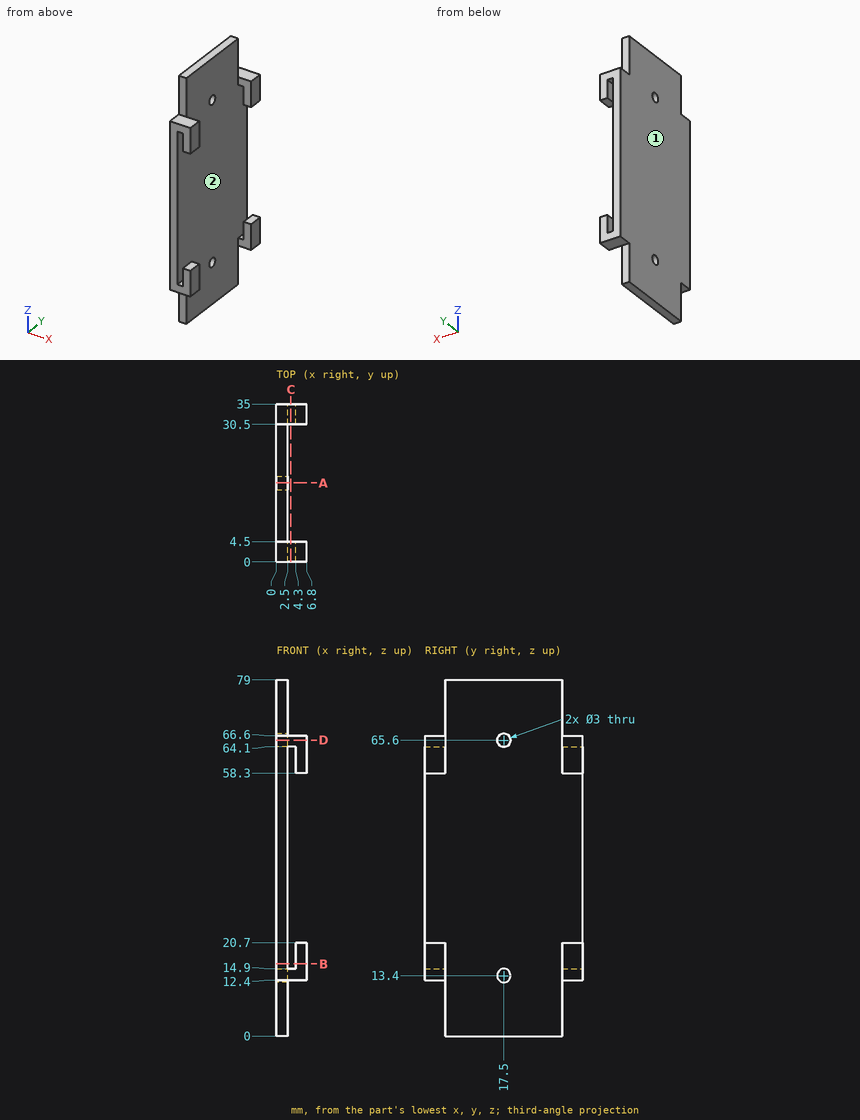
Verification items for this drawing (mm, ordinates from the low corner). Give positions to 0.01 mm unless a question says otherwise; leave off trailing zeros. Loops run counter-clockwise (first coordinate to the right, second up) from the corner with the lowest first, then second, coordinate; pieces in that order, holes last.
1. Cross-section at B-B on z = 16. Record the cut outline in (x, y).
Derived:
outline: (0, 0) - (2.5, 0) - (2.5, 35) - (0, 35) - close; (4.3, 0) - (6.8, 0) - (6.8, 4.5) - (4.3, 4.5) - close; (4.3, 30.5) - (6.8, 30.5) - (6.8, 35) - (4.3, 35) - close
2. Cross-section at D-D on z = 65.6. Record the cut outline in (x, y), and give its area (3 significant figures).
Derived:
outline: (0, 0) - (6.8, 0) - (6.8, 4.5) - (2.5, 4.5) - (2.5, 16) - (0, 16) - close; (0, 19) - (2.5, 19) - (2.5, 30.5) - (6.8, 30.5) - (6.8, 35) - (0, 35) - close
area: 119 mm2
3. Cross-section at A-A on y = 17.5. Record the cut outline in (x, z), and give its area (4 significant figures).
Derived:
outline: (0, 0) - (2.5, 0) - (2.5, 11.9) - (0, 11.9) - close; (0, 14.9) - (2.5, 14.9) - (2.5, 64.1) - (0, 64.1) - close; (0, 67.1) - (2.5, 67.1) - (2.5, 79) - (0, 79) - close
area: 182.5 mm2
4. Cross-section at C-C on x = 3.25. Record the cut outline in (y, z), and give its area (3 significant figures).
Derived:
outline: (0, 12.4) - (4.5, 12.4) - (4.5, 14.9) - (0, 14.9) - close; (0, 64.1) - (4.5, 64.1) - (4.5, 66.6) - (0, 66.6) - close; (30.5, 12.4) - (35, 12.4) - (35, 14.9) - (30.5, 14.9) - close; (30.5, 64.1) - (35, 64.1) - (35, 66.6) - (30.5, 66.6) - close
area: 45.0 mm2
5. Go/stop test with flat-tipped pins: P1, Ø3, axis at y = 30.5, z = 34, coming from the +X side; P2, Ø12, axis at y = 20.5, z = 24, coming from the -X side; P3, Ø0.5, axis at x = 3.5, y = 2.5, coming from the +Z side; P4, Ø2, axis at x = 1.5, z = 8.5, coming from the +Y side. Record where each tip stops, or that it passes through.
Derived:
P1: stops at x = 2.5
P2: stops at x = 0
P3: stops at z = 66.6
P4: stops at y = 30.5
6. Release check for a two-part mould opening along Z. For the marked faces 1 and 2 record: +Z half, -Z half, draft (parallel to the pull), parting line (faces both ways), or undercut.
Derived:
face 1: draft
face 2: undercut
7. Material ranges on probe 1 along X at (y, z) = (1, 19); probe 2 along Y at (x, z) = (1.45, 13.4); probe 3 along Z at (x, y) = (6, 31.5), recorded low to high.
Derived:
probe 1: x = 0 to 2.5, 4.3 to 6.8
probe 2: y = 0 to 16, 19 to 35
probe 3: z = 12.4 to 20.7, 58.3 to 66.6
